from build123d import *

# Parameters (mm, degrees)
SKETCH1_W                                      = 3.275
SKETCH1_H                                      = 3.275
SKETCH1_W_2                                    = 4.6228
SKETCH1_H_2                                    = 4.6228
BOSS_EXTRUDE1_DEPTH                            = 6.35
CBORE_FOR_8_BUTTON_HEAD_CAP_SCREW1_D           = 4.4958
CBORE_FOR_8_BUTTON_HEAD_CAP_SCREW1_CBORE_D     = 8.73252
CBORE_FOR_8_BUTTON_HEAD_CAP_SCREW1_CBORE_DEPTH = 2.7178
CBORE_FOR_8_BUTTON_HEAD_CAP_SCREW2_D           = 4.4958
CBORE_FOR_8_BUTTON_HEAD_CAP_SCREW2_CBORE_D     = 8.73252
CBORE_FOR_8_BUTTON_HEAD_CAP_SCREW2_CBORE_DEPTH = 2.7178


with BuildPart() as part:
    # Sketch1 → Boss-Extrude1 (new body)
    with BuildSketch(Plane(origin=(0, 0, 0), x_dir=(0, 0, -1), z_dir=(1, 0, 0))):
        with BuildLine():
            Line((-83.439, -6.35), (25.4, -6.35))
            ThreePointArc((25.4, -6.35), (31.75, 0), (25.4, 6.35))
            Line((25.4, 6.35), (-83.439, 6.35))
            ThreePointArc((-83.439, 6.35), (-89.789, 0), (-83.439, -6.35))
        make_face()
        Rectangle(SKETCH1_W, SKETCH1_H, mode=Mode.SUBTRACT)
        with Locations((-83.439, 0)):
            Rectangle(SKETCH1_W_2, SKETCH1_H_2, mode=Mode.SUBTRACT)
        with Locations((-58.039, 0)):
            Rectangle(SKETCH1_W_2, SKETCH1_H_2, mode=Mode.SUBTRACT)
        with Locations((-70.739, 0)):
            Rectangle(SKETCH1_W_2, SKETCH1_H_2, mode=Mode.SUBTRACT)
    extrude(amount=BOSS_EXTRUDE1_DEPTH)

    # CBORE for #8 Button Head Cap Screw1 (through all)
    with Locations(Plane(origin=(6.35, 0, 25.4), x_dir=(0, 0, 1), z_dir=(1, 0, 0))):
        with Locations((0, 0), (-50.8, 0)):
            CounterBoreHole(CBORE_FOR_8_BUTTON_HEAD_CAP_SCREW1_D / 2, CBORE_FOR_8_BUTTON_HEAD_CAP_SCREW1_CBORE_D / 2, CBORE_FOR_8_BUTTON_HEAD_CAP_SCREW1_CBORE_DEPTH)

    # CBORE for #8 Button Head Cap Screw2 (through all)
    with Locations(Plane(origin=(0, 0, 70.739), x_dir=(0, 0, -1), z_dir=(-1, 0, 0))):
        with Locations((0, 0)):
            CounterBoreHole(CBORE_FOR_8_BUTTON_HEAD_CAP_SCREW2_D / 2, CBORE_FOR_8_BUTTON_HEAD_CAP_SCREW2_CBORE_D / 2, CBORE_FOR_8_BUTTON_HEAD_CAP_SCREW2_CBORE_DEPTH)


solid = part.part
Model file for the job. Use its own axes, mm. A direction names the side the tool comes from. Give positions to 0.01 mm unless a question says otherwise; leave off trailing zeros. Write each loop counter-clockwise with the first axis right and the second up, starting at its lowest first coordinate (ties: lowest second). Pieces come first, ordered by that corner, then holes. Notation, with made-up numbers: (-25, 9.25) - (7, 9.25) arc R23 ccw to (7, 37.25) - close; hole circle Ø5 at (42, -12). An arc over 180 degrees is marked (long way). Answer as CSV lines item,"result".
1. Band-saw the part on A-A (x = 5). Write the cut outline in (y, z), and give its area (3 significant figures).
Responses:
outline,"(-6.35, -25.4) arc R6.35 ccw to (6.35, -25.4) - (6.35, 83.44) arc R6.35 ccw to (-6.35, 83.44) - close; hole circle Ø8.73 at (0, -25.4); hole circle Ø8.73 at (0, 25.4); hole (-2.31, 55.73) - (2.31, 55.73) - (2.31, 60.35) - (-2.31, 60.35) - close; hole (-2.31, 68.43) - (2.31, 68.43) - (2.31, 73.05) - (-2.31, 73.05) - close; hole (-2.31, 81.13) - (2.31, 81.13) - (2.31, 85.75) - (-2.31, 85.75) - close; hole (-1.64, -1.64) - (1.64, -1.64) - (1.64, 1.64) - (-1.64, 1.64) - close"
area,"1,310 mm2"
2. Band-saw the part on C-C (y = 0). Count the separate pieces of the cut face and the enclosed holes in it, and give its area (3 significant figures).
Responses:
separate pieces,"7"
enclosed holes,"0"
area,"572 mm2"
3. Pin check, flat tips, straight feed: pin 1 (4.5 mm diameter, centred on y = -0.5, z = 24.5, fed in from +X); pin 2 (3.5 mm diameter, centred on x = 2.5, y = -0.5, fed in from -Z); pin 3 (1 mm diameter, centred on x = 3, y = -3.5, fed in from +Z); pin 4 (3 mm diameter, centred on x = 3, y = 4, fed in from +Z). Stop position of each tip, or through.
Responses:
pin 1,"stops at x = 3.63"
pin 2,"stops at z = -31.75"
pin 3,"stops at z = 89.04"
pin 4,"stops at z = 89.28"
4. Band-saw the part on B-B (z = 25.4). Write the cut outline in (x, y).
Responses:
outline,"(0, -6.35) - (6.35, -6.35) - (6.35, -4.37) - (3.63, -4.37) - (3.63, -2.25) - (0, -2.25) - close; (0, 2.25) - (3.63, 2.25) - (3.63, 4.37) - (6.35, 4.37) - (6.35, 6.35) - (0, 6.35) - close"
5. 3-axis set-ups, long thin cutter, end or side, ignore diameter. For faces 3 (the face through (3.632, -1, 23)), 4 (the face through (5, 0, 68.428)), 5 (the face through (0, 0, 30)), 6 (the face through (1.34, -1.312, 66.574)): which of +Z, -Z, +X, -X, +Y, -Y reach the whole face in a straight line?
Responses:
face 3,"+X"
face 4,"+X, -X"
face 5,"+Z, -Z, -X, +Y, -Y"
face 6,"-X"
6. Drill centre lines: L1, parallel to Y at x = 4.85, z = -25.4; L2, parallel to X at y = -1.25, z = 29.5; L3, parallel to Z at x = 5.5, y = 2.25. Where is each one in solid material? Low to high. Write a range as [from, to].
Responses:
L1,"y = [-6.35, -4.37], [4.37, 6.35]"
L2,"x = [0, 3.63]"
L3,"z = [-31.34, -29.14], [-21.66, 21.66], [29.14, 55.73], [60.35, 68.43], [73.05, 81.13], [85.75, 89.38]"
7. Two-plate mould, pull along Z, no slides. Class faces 1 (the face through (3, -6.35, 30)), 2 (the face through (5, 2.311, 71)): +Z half, -Z half, draft (parallel to the pull), parting line (faces both ways), or undercut.
Responses:
face 1,"draft"
face 2,"undercut"
